```python
from build123d import *

# Parameters (mm, degrees)
F1_DEPTH = 2
F3_DEPTH = 1.5


with BuildPart() as f1:
    # F0 (on Front) → F1 (new body)
    with BuildSketch(Plane.XZ):
        with BuildLine():
            Line((-27, 0), (-25, 0))
            ThreePointArc((-25, 0), (0, 25), (25, 0))
            Line((25, 0), (25, -77.667619))
            Line((25, -77.667619), (27, -78.867619))
            Line((27, -78.867619), (27, 0))
            ThreePointArc((27, 0), (0, 27), (-27, 0))
        make_face()
        Polygon((27, -78.867619), (25, -77.667619), (-182.220635, -202), (232.220635, -202), align=None)
        Polygon((-175, -200), (25, -80), (225, -200), align=None, mode=Mode.SUBTRACT)
    extrude(amount=F1_DEPTH)

    # F2 (on Front) → F3 (join, symmetric)
    with BuildSketch(Plane.XZ):
        Polygon((92, -82), (-38, -82), (-193, -212), (-300, -882), (300, -882), (247, -212), align=None)
    extrude(amount=F3_DEPTH, both=True)


solid = f1.part
```
Read the model definition and answer for the solid it produces. Units are mm, in the model's axes. A direction names the side the tool comes from. Give positions to 0.01 mm unless a question says otherwise; leave off trailing zeros. Write each loop counter-clockwise with the first axis right and the second up, starting at its lowest first coordinate (ties: lowest second). Pieces come first, ordered by that corner, then holes. Notation, with made-up numbers: (20, 24) -> (32, 24) arc R36 ccw to (32, 60) -> close; hole circle Ø11 at (76.5, 80). An arc over 180 degrees is marked (long way). Answer in a Markdown table with one row per item.
1) Each of these flat-tipped pins is pushed along its axis until it touches: pin 1 Ø1.6 at (y, z) = (-1.5, -22) entering from -X; pin 2 Ø1.5 at (x, z) = (-4.5, -763) entering from -Y; pin 3 Ø1 at (y, z) = (0.5, -180) entering from +X. Where does it stop, or does it pass through?
Results list:
| item | result |
|---|---|
| pin 1 | x = 25 |
| pin 2 | y = -1.5 |
| pin 3 | x = 209.44 |
2) Section A-A on x = 0 is taken. Give the vertices of the cut face in (y, z), plus the area to 3 significant figures.
Results list:
| item | result |
|---|---|
| outline | (-2, -202) -> (-1.5, -202) -> (-1.5, -882) -> (1.5, -882) -> (1.5, -82) -> (-1.5, -82) -> (-1.5, -92.67) -> (-2, -92.67) -> (-2, -95) -> (-1.5, -95) -> (-1.5, -200) -> (-2, -200) -> close; (-2, 25) -> (0, 25) -> (0, 27) -> (-2, 27) -> close |
| area | 2,410 mm^2 |
3) Section B-B on y = 0.65 is taken. Give the vertices of the cut face in (x, z), plus the area to 3 significant figures.
Results list:
| item | result |
|---|---|
| outline | (-300, -882) -> (300, -882) -> (247, -212) -> (92, -82) -> (-38, -82) -> (-193, -212) -> close |
| area | 385,000 mm^2 |
4) Section D-D on z = -678 is taken. Give the vertices of the cut face in (x, y).
Results list:
| item | result |
|---|---|
| outline | (-267.42, -1.5) -> (283.86, -1.5) -> (283.86, 1.5) -> (-267.42, 1.5) -> close |
5) Determine the mould class of faces 4 (the flat face through (273.87, -0.02, -551.69)), 5 (the flat face through (-70.452, -1.736, -134.939)), 6 (the flat face through (117.13, -1.74, -135.28)) for opening direction Z: released by +Z, released by -Z, zero draft, split by the parting line, or undercut.
Results list:
| item | result |
|---|---|
| face 4 | released by +Z |
| face 5 | undercut |
| face 6 | undercut |
6) Section C-C on x = 173.5 is taken. Give the vertices of the cut face in (y, z), plus the area to 3 significant figures.
Results list:
| item | result |
|---|---|
| outline | (-2, -202) -> (-1.5, -202) -> (-1.5, -882) -> (1.5, -882) -> (1.5, -150.35) -> (-1.5, -150.35) -> (-1.5, -166.77) -> (-2, -166.77) -> (-2, -169.1) -> (-1.5, -169.1) -> (-1.5, -200) -> (-2, -200) -> close |
| area | 2,200 mm^2 |
7) A tool of negligible diameter and unlimited length cuts with its end or side. For faces 1 (the flat face through (26.6, 0, -15.1)), 2 (the cylindrical face through (-0.55, -0.986, 24.994)), 3 (the cylindrical face through (0.594, -0.986, 26.993)), from which of +Z, -Z, +X, -X, +Y, -Y can it reach the whole face along a straight path? Write none if from no direction.
Results list:
| item | result |
|---|---|
| face 1 | +Z, +X, -X, +Y |
| face 2 | +Y, -Y |
| face 3 | +Z, +Y, -Y |
8) Straight lines are drawn through the part: line 1 (Z direction, x = 11, y = -0.1); line 2 (Y direction, x = -225, z = -672.5); line 3 (Z direction, x = 50, y = -0.5). For each, find the intervals that lie inside material, in ascending order. Write a range as [from, to].
Results list:
| item | result |
|---|---|
| line 1 | [-882, -82], [22.45, 24.66] |
| line 2 | [-1.5, 1.5] |
| line 3 | [-882, -82] |
